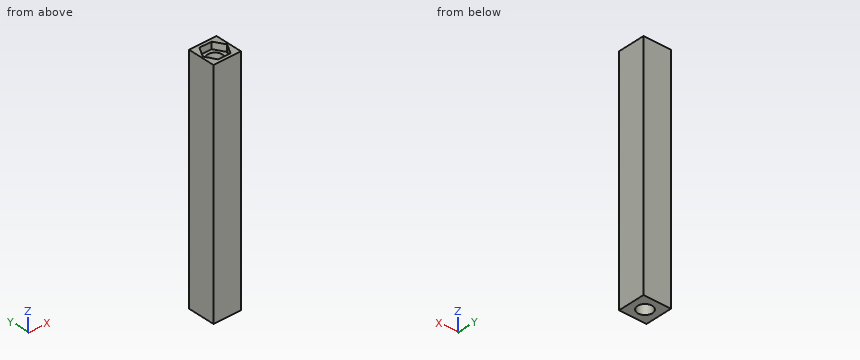
Autodesk Inventor part; units mm, degrees
ref_plane "YZ Plane" through (0, 0, 0) normal (1, 0, 0) x (0, 1, 0)
ref_plane "XZ Plane" through (0, 0, 0) normal (0, 1, 0) x (-1, 0, 0)
ref_plane "XY Plane" through (0, 0, 0) normal (0, 0, 1) x (1, 0, 0)
sketch "Sketch1" plane through (0, 0, 0) normal (0, 0, 1) x (1, 0, 0)
  line L0 (5, -5) -> (5, 5)
  line L1 (-5, -5) -> (5, -5)
  line L2 (-5, 5) -> (-5, -5)
  line L3 (5, 5) -> (-5, 5)
  circle A0 centre (0, 0) radius 3
  line L4 (2.8868, -5) -> (5.7735, 0)
  line L5 (2.8868, -5) -> (5.7735, 0)
  line L6 (-2.8868, -5) -> (2.8868, -5)
  line L7 (-5.7735, 0) -> (-2.8868, -5)
  line L8 (-2.8868, 5) -> (-5.7735, 0)
  line L9 (2.8868, 5) -> (-2.8868, 5)
  line L10 (5.7735, 0) -> (2.8868, 5)
  circle A1 centre (0, 0) radius 2.9998
  line L11 (6.5, -6.5) -> (-6.5, -6.5)
  line L12 (-6.5, -6.5) -> (-6.5, 6.5)
  line L13 (-6.5, 6.5) -> (6.5, 6.5)
  line L14 (6.5, 6.5) -> (6.5, -6.5)
  line L15 (6.5, -6.5) -> (-6.5, 6.5) construction
  line L16 (-6.5, -6.5) -> (6.5, 6.5) construction
  dimension "d0" = 6
  dimension "d7" = 13
  dimension "d8" = 13
extrude "Extrusion1" add sketch "Sketch1" along normal blind 110 contours L1 L4 L0 | L4 L1 L7 L2 L8 L3 L10 L0 | L0 L10 L4 | L10 L3 L0 | L1 L2 L7 | L7 L8 L2 | L8 L2 L3 | A0 | L11 L12 L13 L14
sketch "Sketch2" plane through (0, 0, 110) normal (0, 0, 1) x (1, 0, 0)
  point P0 (0, 0)
sketch "Sketch3" plane through (0, 0, 110) normal (0, 0, 1) x (1, 0, 0)
  circle A0 centre (0, 0) radius 4
  circle A1 centre (0, 0) radius 3
  line L0 (2.8868, -5) -> (5.7735, 0)
  line L1 (5.7735, 0) -> (2.8868, 5)
  line L2 (2.8868, 5) -> (-2.8868, 5)
  line L3 (-2.8868, 5) -> (-5.7735, 0)
  line L4 (-5.7735, 0) -> (-2.8868, -5)
  line L5 (-2.8868, -5) -> (2.8868, -5)
extrude "Extrusion2" cut sketch "Sketch3" against normal blind 3.22 contours A0 | A1 | L5 L4 L3 L2 L1 L0
sketch "Sketch4" plane through (0, 0, 0) normal (0, 0, -1) x (-1, 0, 0)
  circle A0 centre (0, 0) radius 3.5
  dimension "d9" = 7
extrude "Extrusion3" cut sketch "Sketch4" against normal through all
properties part number "plunger"
For this review, take the finished solid that the model builds, in its own axes (mm). Round coordinates to 2 decimals unless told otherwise and drop trailing zeros. Write each loop counter-clockwise with the first axis right and the second up, starting at its lowest first coordinate (ties: lowest second). Pieces come first, ordered by that corner, then holes. Notation, with made-up numbers: (-2.75, 82) - (38.25, 82) arc R29 ccw to (38.25, 106) - close; hole circle Ø6 at (82, -40). An arc over 180 degrees is marked (long way). Answer as a JSON object with one key per item and string values.
1. For pin 1 Ø2 at (x, y) = (-5, 1) entering from -Z, flat-tipped, find the tip position at first contact; note if it passes through.
Response values:
{"pin 1": "stops at z = 0"}
2. To check wall thickness, follow line 1 along Y through (x, z) = (0, 78); line 2 along X through (y, z) = (-2, 47.5); line 3 along Z through (x, y) = (4, -1). State the ranges of each line that lie inside material, in increasing order.
Response values:
{"line 1": "y = -6.5 to -3.5, 3.5 to 6.5", "line 2": "x = -6.5 to -2.87, 2.87 to 6.5", "line 3": "z = 0 to 106.78"}
3. We need section C-C on y = -1.5. Give the boundary of the cut face in (x, z).
Response values:
{"outline": "(-6.5, 0) - (-3.16, 0) - (-3.16, 106.78) - (-4.91, 106.78) - (-4.91, 110) - (-6.5, 110) - close; (3.16, 0) - (6.5, 0) - (6.5, 110) - (4.91, 110) - (4.91, 106.78) - (3.16, 106.78) - close"}
4. We need section A-A on x = 0. Give the boundary of the cut face in (y, z).
Response values:
{"outline": "(-6.5, 0) - (-3.5, 0) - (-3.5, 106.78) - (-5, 106.78) - (-5, 110) - (-6.5, 110) - close; (3.5, 0) - (6.5, 0) - (6.5, 110) - (5, 110) - (5, 106.78) - (3.5, 106.78) - close"}
5. We need section B-B on z = 83. Give the boundary of the cut face in (x, y), then the cut area to 3 significant figures.
Response values:
{"outline": "(-6.5, -6.5) - (6.5, -6.5) - (6.5, 6.5) - (-6.5, 6.5) - close; hole circle Ø7 at (0, 0)", "area": "131 mm2"}
